Can you work these out from the drawing? Everything is in mm from the part's minimum corner. Round coordinates to 2 decimals unless told otherwise and drop trailing zeros. Write each loop counter-clockwise with the first axis right and the second up, starting at its lowest first coordinate (ties: lowest second). Pieces come first, ordered by that corner, then holes. Notation, with made-up numbers: (54.5, 28) -> (72.5, 28) arc R8 cw to (72.5, 38) -> close; hole circle Ø9 at (47.25, 14). An arc over 180 degrees is marked (long way). Put each result on its own line as item: value. Start each with the question number.
1. For pin 1 (3 mm diameter, centred on x = 33.02, z = 33.02, fed in from -Y), with a flat end and sliding along its axis, tell me the tip position at first contact or that it passes through.
2. Suppose I cut it at B-B (y = 4.4). Please give me the cut outline in (x, z) (3 decimals).
3. Suppose I cut it at C-C (x = 14). Please give me the cut outline in (y, z).
4. We'd pull the mould along Z, two halves only. Please class the marked faces 1, 2 and 3: +Z half, -Z half, draft (parallel to the pull), parting line (faces both ways), or undercut.
5. Suppose I cut it at A-A (z = 19.05). Please give me the cut outline in (x, y).
6. I need wall thicknesses on probe 1 along Z at (x, y) = (19.5, 3.65); probe 2 along X at (y, z) = (2.1, 19); probe 3 along X at (y, z) = (2.3, 34.5). Which ranges of each line are inside material? Lowest first, please. Write a range as from..to.
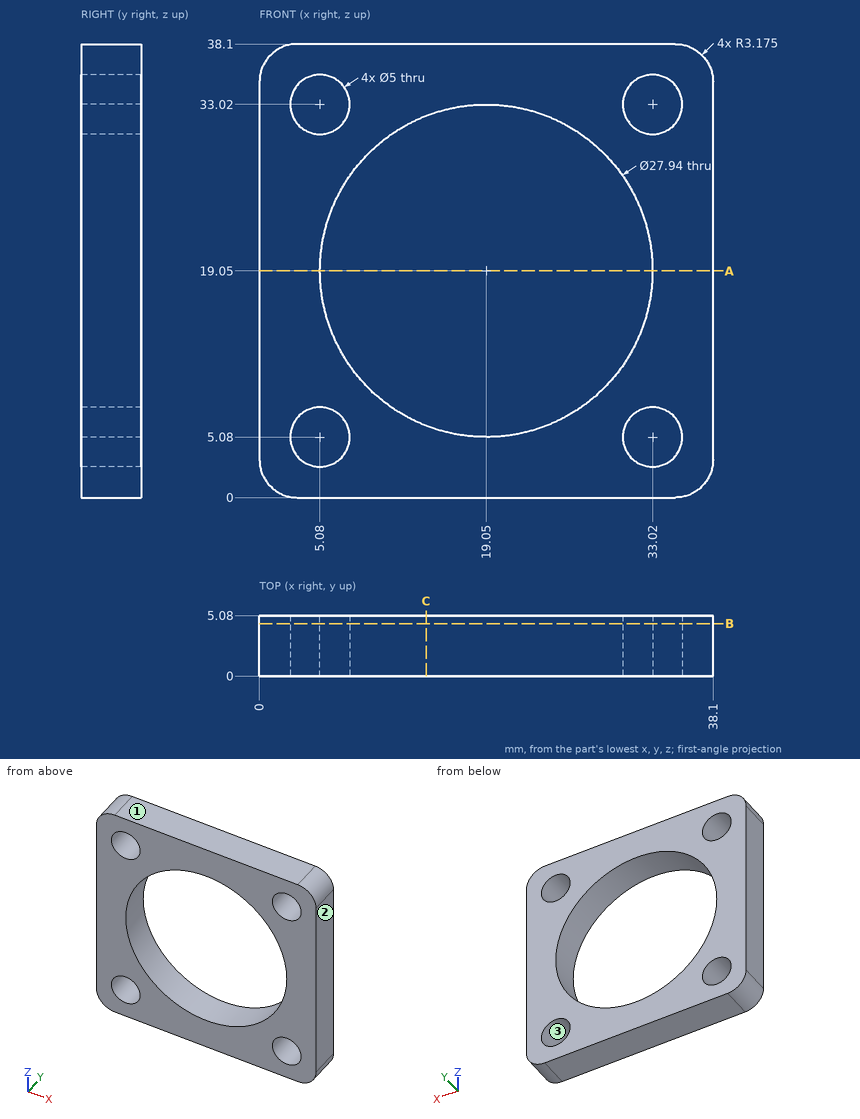
Verdict:
1. pin 1: passes through
2. outline: (0, 3.175) arc R3.175 ccw to (3.175, 0) -> (34.925, 0) arc R3.175 ccw to (38.1, 3.175) -> (38.1, 34.925) arc R3.175 ccw to (34.925, 38.1) -> (3.175, 38.1) arc R3.175 ccw to (0, 34.925) -> close; hole circle Ø5 at (5.08, 5.08); hole circle Ø5 at (5.08, 33.02); hole circle Ø27.94 at (19.05, 19.05); hole circle Ø5 at (33.02, 5.08); hole circle Ø5 at (33.02, 33.02)
3. outline: (0, 0) -> (5.08, 0) -> (5.08, 6.02) -> (0, 6.02) -> close; (0, 32.08) -> (5.08, 32.08) -> (5.08, 38.1) -> (0, 38.1) -> close
4. face 1: +Z half
4. face 2: draft
4. face 3: undercut
5. outline: (0, 0) -> (5.08, 0) -> (5.08, 5.08) -> (0, 5.08) -> close; (33.02, 0) -> (38.1, 0) -> (38.1, 5.08) -> (33.02, 5.08) -> close
6. probe 1: z = 0..5.09, 33.01..38.1
6. probe 2: x = 0..5.08, 33.02..38.1
6. probe 3: x = 0..3.07, 7.09..31.01, 35.03..38.1
